```python
from build123d import *

# Parameters (mm, degrees)
SKETCH1_R           = 5.75
BOSS_EXTRUDE1_DEPTH = 3
BOSS_EXTRUDE2_DEPTH = 0.15
CIRPATTERN1_COUNT   = 2
SKETCH5_R           = 2.5
CUT_EXTRUDE1_DEPTH  = 65.479328162
CHAMFER1_SIZE       = 1


with BuildPart() as part:
    # Sketch1 → Boss-Extrude1 (new, symmetric)
    with BuildSketch(Plane(origin=(0, 0, 0), x_dir=(1, 0, 0), z_dir=(0, 1, 0))):
        with Locations(Location((0, 0, 0), (0, 0, 270))):
            Circle(SKETCH1_R)
    extrude(amount=BOSS_EXTRUDE1_DEPTH, both=True)

    # Sketch4 → Boss-Extrude2 (add, symmetric)
    with BuildSketch(Plane(origin=(0, 0, 0), x_dir=(0.9743700647852352, -0.22495105434386534, 0), z_dir=(-0.2249510543438653, -0.9743700647852351, 0))):
        with BuildLine():
            Line((-2.09695858, 4.179050657), (-4.927774709, 8.201975805))
            Line((-4.927774709, 8.201975805), (-4.927774709, 60.5))
            ThreePointArc((-4.927774709, 60.5), (-4.049095053, 62.621320344), (-1.927774709, 63.5))
            Line((-1.927774709, 63.5), (0.385917788, 63.5))
            ThreePointArc((0.385917788, 63.5), (3.272130568, 62.582863675), (5.099523115, 60.167910314))
            add(Edge.make_bspline(
                [(3.648123834, 4.179050657), (11.246463355, 22.537150452), (11.557411768, 41.917565493), (5.099523115, 60.167910314)],
                knots=[0, 0, 0, 0, 0.942591792, 0.942591792, 0.942591792, 0.942591792], degree=3))
            Line((3.648123834, 4.179050657), (-2.09695858, 4.179050657))
        make_face()
    boss_extrude2 = extrude(amount=BOSS_EXTRUDE2_DEPTH, both=True)

    # CirPattern1: Boss-Extrude2 ×2 about axis
    cirpattern1_axis = Axis((0, -3, 0), (0, 1, 0))
    for i in range(1, CIRPATTERN1_COUNT):
        add(boss_extrude2.rotate(cirpattern1_axis, i * 360 / CIRPATTERN1_COUNT))

    # Sketch5 → Cut-Extrude1 (cut, through all)
    with BuildSketch(Plane.XZ.offset(3)):
        with Locations(Location((0, 0, 0), (0, 0, 270))):
            Circle(SKETCH5_R)
    extrude(amount=-CUT_EXTRUDE1_DEPTH, mode=Mode.SUBTRACT)

    # Chamfer1
    chamfer1_edges = [part.edges().sort_by_distance(p)[0] for p in [
        (0, -3, 2.5),
    ]]
    chamfer(chamfer1_edges, length=CHAMFER1_SIZE)


solid = part.part
```
Model file for the job. Use its own axes, mm. A direction names the side the tool comes from. Coordinates: 2 decimals unless noted, no trailing zeros. Write each loop counter-clockwise with the first axis right and the second up, starting at its lowest first coordinate (ties: lowest second). Pieces come first, ordered by that corner, then holes. Notation, with made-up numbers: (33, -25) - (91, -25) arc R19 ccw to (91, -11) - close; hole circle Ø11 at (59, 69). An arc over 180 degrees is marked (long way). Use a Markdown table: item, result. Add a question column.
Item 1: Two-plate mould, pull along Z, no slides. Class faces 3 (the face through (1.58, -0.21, 34.37)), 4 (the face through (-2.44, 0.46, 0.54)): pulls with the +Z half, pulls with the -Z half, needs draft (parallel to the pull), parting line crosses it, or undercut.
Item 2: 3-axis set-ups, long thin cutter, end or side, ignore diameter. For faces 1 (the face through (1.727, 0.042, 5.484)), 2 (the face through (0, -3, 4)): which of +Z, -Z, +X, -X, +Y, -Y reach the whole face in a straight line?
Item 3: Drop flat-ended pins along their axis: pin 1 (3 mm diameter, centred on y = 2, z = 22.5, fed in from -X); pin 2 (8 mm diameter, centred on x = -2, z = -12, fed in from +Y); pin 3 (4 mm diameter, centred on x = -7.5, z = 25, fed in from -Y). Give the stop position or say it passes through.
Item 4: Band-saw the part on A-A, the plane z = 0. Write the cut outline in (x, y).
Item 5: Drill centre lines: line 1 along X through (y, z) = (-0.7, 0); line 2 along Y through (x, z) = (-3.5, -55); line 3 along Y through (x, z) = (7.5, 19.5). Where is each one in solid material? Low to high.
A:
| question | item | result |
|---|---|---|
| 1 | face 3 | needs draft |
| 1 | face 4 | undercut |
| 2 | face 1 | none |
| 2 | face 2 | +Z, -Z, +X, -X, -Y |
| 3 | pin 1 | stops at x = -4.84 |
| 3 | pin 2 | stops at y = 0.62 |
| 3 | pin 3 | passes through |
| 4 | outline | (-5.75, -3) - (-3.5, -3) - (-2.5, -2) - (-2.5, 3) - (-5.75, 3) - close; (2.5, -2) - (3.5, -3) - (5.75, -3) - (5.75, 3) - (2.5, 3) - close |
| 5 | line 1 | x = -5.75 to -2.5, 2.5 to 5.75 |
| 5 | line 2 | y = -0.96 to -0.65 |
| 5 | line 3 | y = -1.89 to -1.58 |
